Input: part model. Units: mm. Frame: model coordinates. A direction names the side the tool comes from. Give positions to 0.01 mm unless a question says otherwise; leave off trailing zeros. Write each loop counter-clockwise with the first axis right and the second up, starting at its lowest first coordinate (ties: lowest second). Pieces come first, ordered by that corner, then holes. Notation, with made-up numbers: (-11, 76.25) - (35, 76.25) arc R20 ccw to (35, 86.25) - close; hole circle Ø11 at (-8, 57). An arc over 180 degrees is marked (long way). Answer as a JSON object with one key per item and string values. Group by question number.
from build123d import *

# Parameters (mm, degrees)
F0_W     = 500
F0_H     = 5
F1_DEPTH = 500
F2_W     = 500
F2_H     = 4.9999952316
F3_DEPTH = 500
F4_W     = 500
F4_H     = 5
F5_DEPTH = 500
F6_W     = 5
F6_H     = 490.0000047684
F6_W_2   = 4.9999952316
F7_DEPTH = 500
F8_R     = 100
F9_DEPTH = 301


with BuildPart() as f1:
    # F0 (on Top) → F1 (new body)
    with BuildSketch(Plane.XY):
        Rectangle(F0_W, F0_H)
    extrude(amount=F1_DEPTH)

    # F2 (on face) → F3 (join)
    with BuildSketch(Plane.XZ.offset(2.5)):
        with Locations((0, 497.5000023842)):
            Rectangle(F2_W, F2_H)
    extrude(amount=F3_DEPTH)

    # F4 (on face) → F5 (join)
    with BuildSketch(Plane.XZ.offset(2.5)):
        with Locations((0, 2.5)):
            Rectangle(F4_W, F4_H)
    extrude(amount=F5_DEPTH)

    # F6 (on face) → F7 (join)
    with BuildSketch(Plane.XZ.offset(2.5)):
        with Locations((247.5, 250.0000023842)):
            Rectangle(F6_W, F6_H)
        with Locations((-247.5000023842, 250.0000023842)):
            Rectangle(F6_W_2, F6_H)
    extrude(amount=F7_DEPTH)

    # F8 (on Right) → F9 (cut, symmetric)
    with BuildSketch(Plane.YZ):
        with Locations((-247.5, 150)):
            Circle(F8_R)
    extrude(amount=F9_DEPTH, both=True, mode=Mode.SUBTRACT)


solid = f1.part
1) Cut plane B-B on z = 150. Return the cut outline in (x, y).
2) Cut plane C-C on x = -219.5. Return the cut outline in (y, z).
3) Pin query (flat end, axial travel): P1, Ø10, axis at x = -36, z = 155.5, coming from the -Y side. Return the tip coordinate at first contact, or that it passes through.
4) Line query: line 1 along Z through (x, y) = (248, -247.5); line 2 along X through (y, z) = (-58, 185); line 3 along Z through (x, y) = (138, -100). Output: solid intervals per line, ascending. Write a range as from..to.
5) Mould query, pull axis X, two halves, no side actions, for faces 1 (the face through (-3, -249, 495)), 2 (the face through (-3, 2.5, 246)), 3 (the face through (245, -249, 301)), 4 (the face through (250, -246, 302)). Classes: +X half, -X half, draft (parallel to the pull), parting line (faces both ways), or undercut.
6) Cut plane A-A on y = -247.5. Return the cut outline in (x, z), and give its area (3 significant figures).
7) Reachability of faces 5 (the face through (-3, -246, 500)), 6 (the face through (-245, -249, 301)) from +Z, -Z, +X, -X, +Y, -Y: full face, straight path, thin tool, end or side. Return the list, or none.
8) Cut plane D-D on z = 85. Return the cut outline in (x, y), and give its area (3 significant figures).
Filled in:
{
 "1": {"outline": "(-250, -502.5) - (-245, -502.5) - (-245, -347.5) - (-250, -347.5) - close; (-250, -147.5) - (-245, -147.5) - (-245, -2.5) - (245, -2.5) - (245, -147.5) - (250, -147.5) - (250, 2.5) - (-250, 2.5) - close; (245, -502.5) - (250, -502.5) - (250, -347.5) - (245, -347.5) - close"},
 "2": {"outline": "(-502.5, 0) - (2.5, 0) - (2.5, 500) - (-502.5, 500) - (-502.5, 495) - (-2.5, 495) - (-2.5, 5) - (-502.5, 5) - close"},
 "3": {"P1": "stops at y = -2.5"},
 "4": {"line 1": "z = 0..50, 250..500", "line 2": "x = -250..-245, 245..250", "line 3": "z = 0..5, 495..500"},
 "5": {"face 1": "undercut", "face 2": "draft", "face 3": "undercut", "face 4": "+X half"},
 "6": {"outline": "(-250, 0) - (250, 0) - (250, 50) - (245, 50) - (245, 5) - (-245, 5) - (-245, 50) - (-250, 50) - close; (-250, 250) - (-245, 250) - (-245, 495) - (245, 495) - (245, 250) - (250, 250) - (250, 500) - (-250, 500) - close", "area": "7,900 mm²"},
 "7": {"face 5": "+Z, +X, -X, +Y, -Y", "face 6": "-Y"},
 "8": {"outline": "(-250, -502.5) - (-245, -502.5) - (-245, -323.49) - (-250, -323.49) - close; (-250, -171.51) - (-245, -171.51) - (-245, -2.5) - (245, -2.5) - (245, -171.51) - (250, -171.51) - (250, 2.5) - (-250, 2.5) - close; (245, -502.5) - (250, -502.5) - (250, -323.49) - (245, -323.49) - close", "area": "5,980 mm²"}
}
